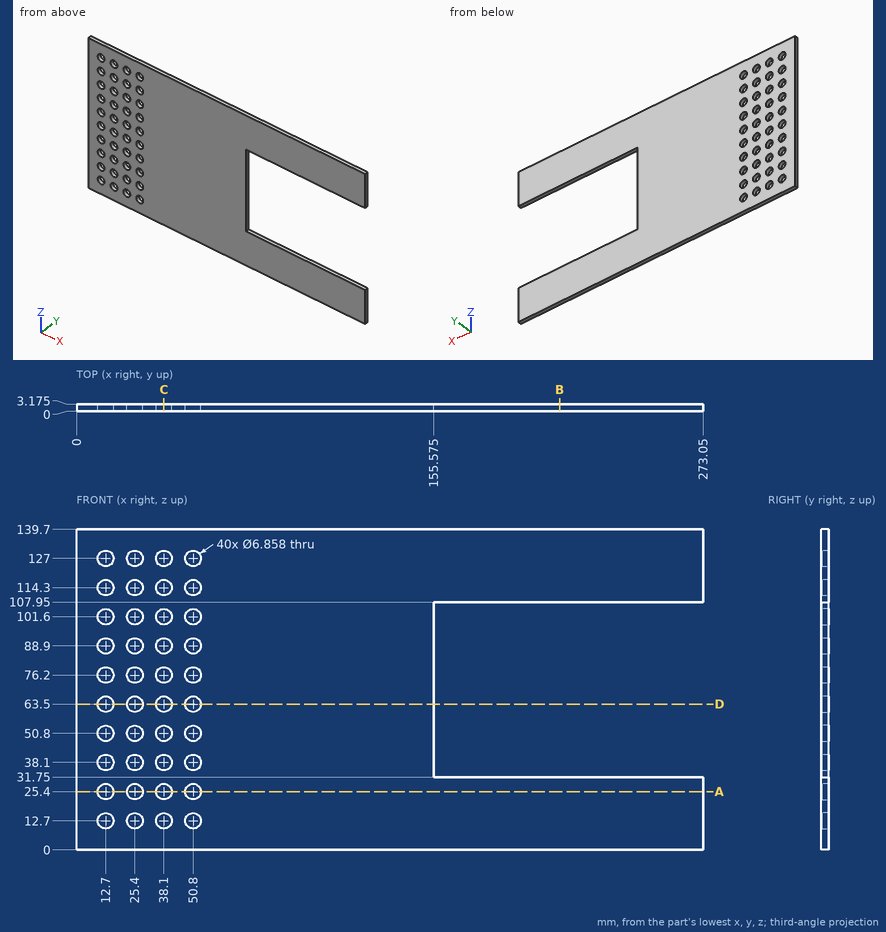
Check sheet for the drawn part. Datum: minimum x, y, z corner. Units: mm. Round coordinates to 2 decimals unless told otherwise and drop trailing zeros. Order: outer loops, then holes, each group sorted by start corner. A loop starts at its lowest first (then second) coordinate and runs counter-clockwise, first axis right, second up.
(1) Cross-section at B-B, the plane x = 210.5. Enter the section's corners in (y, z) (3 decimals), and give its area (3 significant figures).
(2) Cross-section at D-D, the plane z = 63.5. Enter the section's corners in (x, y) (3 decimals), and give its area (3 significant figures).
(3) Cross-section at A-A, the plane z = 25.4. Enter the section's corners in (x, y) (3 decimals).
(4) Cross-section at C-C, the plane x = 38.1. State how many separate pieces and enclosed holes the cut face has, and give its area (3 significant figures).
(5) Scan lines: probe 1 along X at (y, z) = (1.5, 12.7); probe 2 along X at (y, z) = (0.95, 101.6) (3 decimals); probe 3 along Z at (x, y) = (164, 2.6). Record each from-to range of solid material in increasing order.
Check sheet entries:
1. outline: (0, 0) - (3.175, 0) - (3.175, 31.75) - (0, 31.75) - close; (0, 107.95) - (3.175, 107.95) - (3.175, 139.7) - (0, 139.7) - close
1. area: 202 mm2
2. outline: (0, 0) - (9.271, 0) - (9.271, 3.175) - (0, 3.175) - close; (16.129, 0) - (21.971, 0) - (21.971, 3.175) - (16.129, 3.175) - close; (28.829, 0) - (34.671, 0) - (34.671, 3.175) - (28.829, 3.175) - close; (41.529, 0) - (47.371, 0) - (47.371, 3.175) - (41.529, 3.175) - close; (54.229, 0) - (155.575, 0) - (155.575, 3.175) - (54.229, 3.175) - close
2. area: 407 mm2
3. outline: (0, 0) - (9.271, 0) - (9.271, 3.175) - (0, 3.175) - close; (16.129, 0) - (21.971, 0) - (21.971, 3.175) - (16.129, 3.175) - close; (28.829, 0) - (34.671, 0) - (34.671, 3.175) - (28.829, 3.175) - close; (41.529, 0) - (47.371, 0) - (47.371, 3.175) - (41.529, 3.175) - close; (54.229, 0) - (273.05, 0) - (273.05, 3.175) - (54.229, 3.175) - close
4. separate pieces: 11
4. enclosed holes: 0
4. area: 226 mm2
5. probe 1: x = 0 to 9.27, 16.13 to 21.97, 28.83 to 34.67, 41.53 to 47.37, 54.23 to 273.05
5. probe 2: x = 0 to 9.271, 16.129 to 21.971, 28.829 to 34.671, 41.529 to 47.371, 54.229 to 155.575
5. probe 3: z = 0 to 31.75, 107.95 to 139.7
